from build123d import *

# Parameters (mm, degrees)
BOSS_EXTRUDE1_DEPTH                                  = 30
CSK_FOR_M4_HEX_SOCKET_COUNTERSUNK_CAP_SC_D           = 4.5
CSK_FOR_M4_HEX_SOCKET_COUNTERSUNK_CAP_SC_CSINK_D     = 8.96
CSK_FOR_M4_HEX_SOCKET_COUNTERSUNK_CAP_SC_CSINK_ANGLE = 90


with BuildPart() as part:
    # Sketch2 → Boss-Extrude1 (new body)
    with BuildSketch(Plane.XY):
        Polygon((-13, 0), (13, 0), (13, 7.5), (11.5, 9), (5.15, 9), (8.15, 6), (-8.15, 6), (-5.15, 9), (-11.5, 9), (-13, 7.5), align=None)
    extrude(amount=BOSS_EXTRUDE1_DEPTH)

    # CSK for M4 Hex Socket Countersunk Cap Screw1 (through all)
    with Locations(Plane(origin=(0, 6, 0), x_dir=(1, 0, 0), z_dir=(0, 1, 0))):
        with Locations((0, -22.5), (0, -7.5)):
            CounterSinkHole(CSK_FOR_M4_HEX_SOCKET_COUNTERSUNK_CAP_SC_D / 2, CSK_FOR_M4_HEX_SOCKET_COUNTERSUNK_CAP_SC_CSINK_D / 2, counter_sink_angle=CSK_FOR_M4_HEX_SOCKET_COUNTERSUNK_CAP_SC_CSINK_ANGLE)


solid = part.part
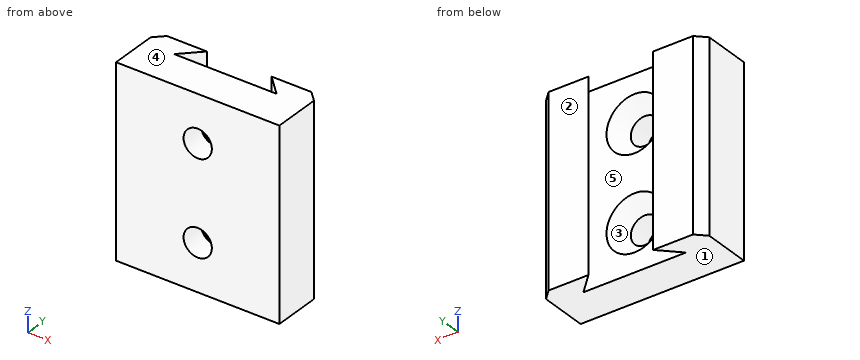
The listing builds one solid part. Answer for the finished solid, in the listing's coordinates (mm). Face numbers are marked on the shaded views. A direction names the side the tool comes from. Give positions to 0.01 mm unless a question says otherwise; leave off trailing zeros. Write each loop counter-clockwise with the first axis right and the second up, starting at its lowest first coordinate (ties: lowest second). Pieces come first, ordered by that corner, then holes.
1) Section A-A (x = 0) is taken. Write down the section's boundary in (y, z), and give its area (3 significant figures).
2) Find the intervals of material crossed by L1, parallel to Z at x = 0, y = 2.3; L2, parallel to X at y = 2.6, z = 22.5; L3, parallel to Y at x = 6, z = 28.5, in increasing order.
3) Section C-C (z = 7.5) is taken. Write down the section's boundary in (x, y).
4) For a pull along Z with two mould halves and no side action, classify the marked faces 1, 2 and 3 as pulls with the +Z half, pulls with the -Z half, needs draft (parallel to the pull), parting line crosses it, or undercut.
5) Given P1, Ø6, axis at x = 0, z = 7.5, coming from the +Y side; P2, Ø1.5, axis at x = 3.5, z = 17.5, coming from the +Y side, each flat-ended and moving along its own axis, determine where each tip first touches the part or whether it passes through.
6) Section B-B (y = 8.5) is taken. Write down the section's boundary in (x, z).
7) Section D-D (y = 5.25) is taken. Write down the section's boundary in (x, z).
8) A tool of negligible diameter and unlimited length cuts with its end or side. For the marked faces 4 and 5, from which of +Z, -Z, +X, -X, +Y, -Y can it reach the whole face along a straight path? Write none if from no direction.
Response:
1. outline: (0, 0) - (6, 0) - (6, 3.02) - (3.77, 5.25) - (0, 5.25) - close; (0, 9.75) - (3.77, 9.75) - (6, 11.98) - (6, 18.02) - (3.77, 20.25) - (0, 20.25) - close; (0, 24.75) - (3.77, 24.75) - (6, 26.98) - (6, 30) - (0, 30) - close
1. area: 116 mm2
2. L1: z = 0 to 5.25, 9.75 to 20.25, 24.75 to 30
2. L2: x = -13 to -2.25, 2.25 to 13
2. L3: y = 0 to 6, 8.15 to 9
3. outline: (-13, 0) - (-2.25, 0) - (-2.25, 3.77) - (-4.48, 6) - (-8.15, 6) - (-5.15, 9) - (-11.5, 9) - (-13, 7.5) - close; (2.25, 0) - (13, 0) - (13, 7.5) - (11.5, 9) - (5.15, 9) - (8.15, 6) - (4.48, 6) - (2.25, 3.77) - close
4. face 1: pulls with the -Z half
4. face 2: needs draft
4. face 3: undercut
5. P1: stops at y = 4.52
5. P2: stops at y = 6
6. outline: (-12, 0) - (-5.65, 0) - (-5.65, 30) - (-12, 30) - close; (5.65, 0) - (12, 0) - (12, 30) - (5.65, 30) - close
7. outline: (-13, 0) - (13, 0) - (13, 30) - (-13, 30) - close; hole circle Ø7.46 at (0, 7.5); hole circle Ø7.46 at (0, 22.5)
8. face 4: +Z, +X, -X, +Y, -Y
8. face 5: +Z, -Z
